Autodesk Inventor part; units mm, degrees
ref_plane "YZ Plane" through (0, 0, 0) normal (1, 0, 0) x (0, 1, 0)
ref_plane "XZ Plane" through (0, 0, 0) normal (0, 1, 0) x (-1, 0, 0)
ref_plane "XY Plane" through (0, 0, 0) normal (0, 0, 1) x (1, 0, 0)
sketch "Sketch1" plane through (0, 0, 0) normal (0, 0, 1) x (1, 0, 0)
  line L0 (-15.9951, 9.4971) -> (34.8049, 9.4971)
  line L1 (34.8049, 9.4971) -> (34.8049, -41.3029)
  line L2 (34.8049, -41.3029) -> (-15.9951, -41.3029)
  line L3 (-15.9951, -41.3029) -> (-15.9951, 9.4971)
  point P0 (0, 0)
  dimension "d0" = 50.8
  dimension "d1" = 50.8
extrude "Extrusion1" add sketch "Sketch1" along normal blind 5.08
ref_plane "Work Plane1" through (0, 0, 132.08) normal (0, 0, 1) x (1, 0, 0)
sketch "Sketch2" plane through (0, 0, 5.08) normal (0, 0, 1) x (1, 0, 0)
  point P0 (0, 0)
sketch "Sketch3" plane through (0, 0, 132.08) normal (0, 0, 1) x (1, 0, 0)
  line L0 (34.8049, 9.4971) -> (-15.9951, 9.4971)
  line L1 (-15.9951, -41.3029) -> (34.8049, -41.3029)
  line L2 (-15.9951, 9.4971) -> (34.8049, -41.3029) construction
  line L3 (34.8049, 9.4971) -> (-15.9951, -41.3029) construction
  circle A0 centre (9.4049, -15.9029) radius 5.715
  point P0 (0, 0)
  dimension "d5" = 11.43
loft "Loft1" add profiles "Sketch3" section 1 edges at (9.4049, 9.4971, 5.08) (-15.9951, -15.9029, 5.08) (9.4049, -41.3029, 5.08) (34.8049, -15.9029, 5.08)
sketch "Sketch4" plane through (9.4049, -15.9029, 132.08) normal (0, 0, 1) x (1, 0, 0)
  circle A0 centre (0, 0) radius 5.3975
  point P0 (-9.4049, 15.9029)
  dimension "d11" = 10.795
extrude "Extrusion2" cut sketch "Sketch4" against normal blind 127
properties part number "arrowadaptor"
Build history of the part. All positions in model axes, mm. Round coordinates to 2 decimals unless told otherwise and drop trailing zeros.
1) Mould opens along X. For faces 1 (the cylindrical face through (14.553, -14.282, 69.469)), 2 (the flat face through (10, -41.303, 3)), 3 (the flat face through (9, -16, 5.08)), 4 (the flat face through (34.805, -16, 3)) say: +X half, -X half, draft (parallel to the pull), parting line (faces both ways), or undercut.
2) Drill centre lines: probe 1 along Y at (x, z) = (8, 105); probe 2 along X at (y, z) = (-14.5, 88); probe 3 along Y at (x, z) = (13, 78). Where is each one in solid material? Low to high.
3) Pin check, flat tips, straight feed: pin 1 (3 mm diameter, centred on x = -3, z = 16.5, fed in from -Y); pin 2 (6 mm diameter, centred on x = -7.5, z = 31.5, fed in from +Y); pin 3 (4 mm diameter, centred on y = -7.5, z = 74, fed in from -X). Stop position of each tip, or through.
Ans:
1. face 1: undercut
1. face 2: draft
1. face 3: undercut
1. face 4: +X half
2. probe 1: y = -25.78 to -21.11, -10.69 to -6.02
2. probe 2: x = -3.13 to 4.19, 14.62 to 21.94
2. probe 3: y = -29.93 to -19.93, -11.88 to -1.88
3. pin 1: stops at y = -39.73
3. pin 2: stops at y = 5.68
3. pin 3: stops at x = -5.34
